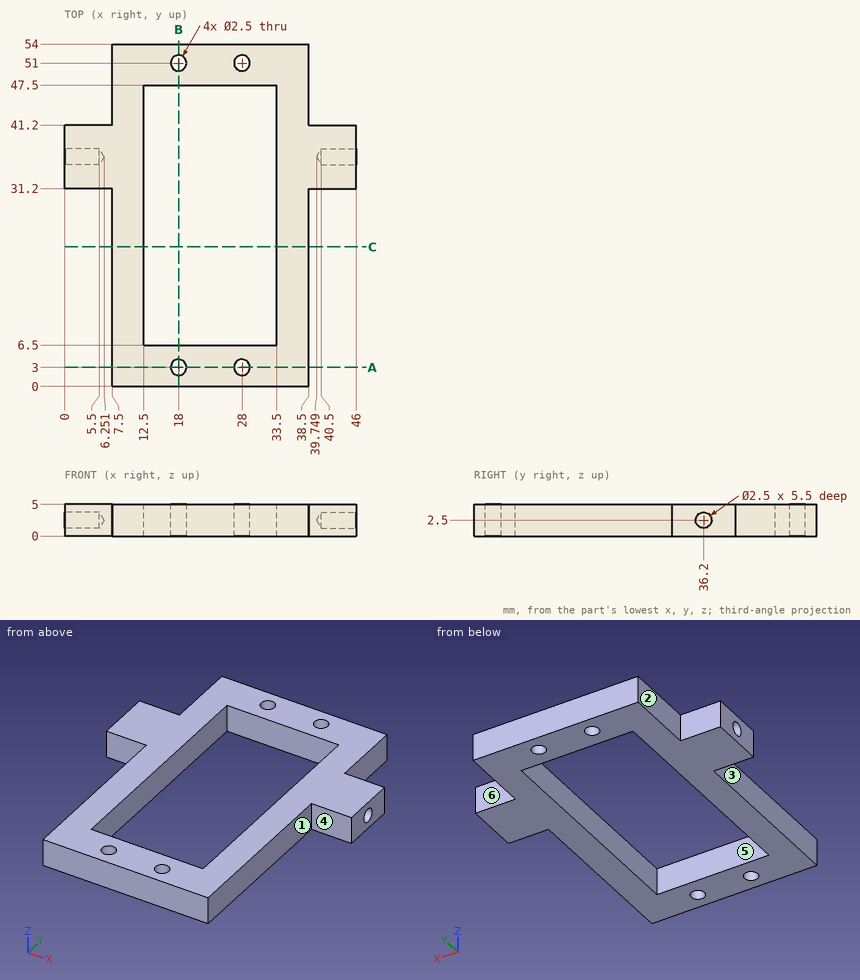
Source: three-view drawing plus pictorial views. Frame: mm from the lowest corner of the part. A direction names the side the tool comes from. Coordinates: 2 decimals unless noted, no trailing zeros. Write each loop counter-clockwise with the first axis right and the second up, starting at its lowest first coordinate (ties: lowest second). Pieces come first, ordered by that corner, then holes. Notation, with made-up numbers: (-38, 47.5) - (-15, 47.5) arc R23 ccw to (-15, 62.5) - close; hole circle Ø9 at (79.5, 19). An arc over 180 degrees is marked (long way). Return JSON: item names as keys, results as strings.
Item 1: Section query B-B (x = 18). Output: boundary loops of the cut face in (y, z), and give its area (3 significant figures).
Completed:
{"outline": "(0, 0) - (1.75, 0) - (1.75, 5) - (0, 5) - close; (4.25, 0) - (6.5, 0) - (6.5, 5) - (4.25, 5) - close; (47.5, 0) - (49.75, 0) - (49.75, 5) - (47.5, 5) - close; (52.25, 0) - (54, 0) - (54, 5) - (52.25, 5) - close", "area": "40.0 mm2"}
Item 2: Section query C-C (y = 22). Output: boundary loops of the cut face in (x, z), and give its area (3 significant figures).
Completed:
{"outline": "(7.5, 0) - (12.5, 0) - (12.5, 5) - (7.5, 5) - close; (33.5, 0) - (38.5, 0) - (38.5, 5) - (33.5, 5) - close", "area": "50.0 mm2"}
Item 3: Pull-direction query (Y, two-part tool) for the marked faces 4, 5 and 6; classes: +Y half, -Y half, draft (parallel to the pull), parting line (faces both ways), or undercut.
Completed:
{"face 4": "-Y half", "face 5": "undercut", "face 6": "+Y half"}
Item 4: Reachability of the marked faces 1, 2 and 3 from +Z, -Z, +X, -X, +Y, -Y: full face, straight path, thin tool, end or side. Return the list, or none.
Completed:
{"face 1": "+Z, -Z, +X, -Y", "face 2": "+Z, -Z, -X, +Y", "face 3": "+Z, -Z, -X, -Y"}
Item 5: Section query A-A (y = 3). Output: boundary loops of the cut face in (x, z).
Completed:
{"outline": "(7.5, 0) - (16.75, 0) - (16.75, 5) - (7.5, 5) - close; (19.25, 0) - (26.75, 0) - (26.75, 5) - (19.25, 5) - close; (29.25, 0) - (38.5, 0) - (38.5, 5) - (29.25, 5) - close"}
Item 6: Pin query (flat end, axial travel): pin 1 Ø4 at (x, y) = (28, 3) entering from -Z; pin 2 Ø2.5 at (x, z) = (5.5, 1.5) entering from +Y; pin 3 Ø1 at (y, z) = (28.5, 4) entering from -X; pin 4 Ø2.5 at (y, z) = (14.5, 2) entering from +X. Return the tip coordinate at first contact, or that it passes through.
Completed:
{"pin 1": "stops at z = 0", "pin 2": "stops at y = 41.2", "pin 3": "stops at x = 7.5", "pin 4": "stops at x = 38.5"}
Item 7: Line query: L1, parallel to Y at x = 28, z = 3.9; L2, parallel to X at y = 12.5, z = 3.9; L3, parallel to X at y = 31.5, z = 2.9. Output: solid intervals per line, ascending.
Completed:
{"L1": "y = 0 to 1.75, 4.25 to 6.5, 47.5 to 49.75, 52.25 to 54", "L2": "x = 7.5 to 12.5, 33.5 to 38.5", "L3": "x = 0 to 12.5, 33.5 to 46"}
